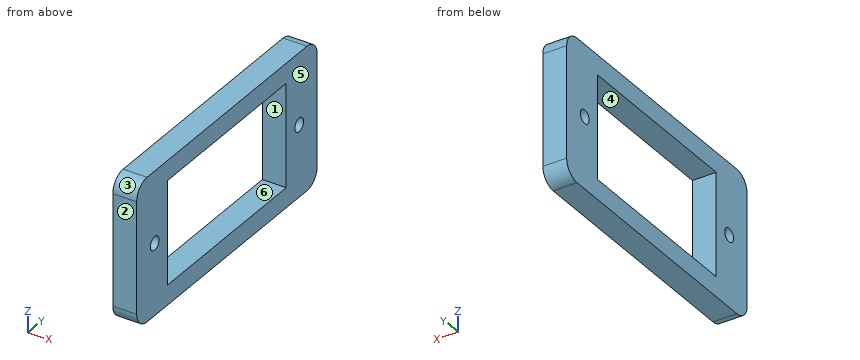
```python
from build123d import *

# Parameters (mm, degrees)
ESBO_O1_W                = 18
ESBO_O1_H                = 35
RESSALTO_EXTRUS_O1_DEPTH = 3
CORTE_EXTRUS_O1_REACH    = 21.906
ESBO_O2_W                = 13
ESBO_O2_H                = 23
CORTE_EXTRUS_O2_REACH    = 21.906
ESBO_O3_R                = 0.85
FILETE1_R                = 2


with BuildPart() as part:
    # Esboço1 → Ressalto-extrusão1 (new body)
    with BuildSketch(Plane(origin=(0, 0, 0), x_dir=(0, 0, -1), z_dir=(1, 0, 0))):
        Rectangle(ESBO_O1_W, ESBO_O1_H)
    extrude(amount=RESSALTO_EXTRUS_O1_DEPTH)

    # Esboço2 → Corte-extrusão1 (cut, up to next)
    with BuildSketch(Plane(origin=(3, 0, 0), x_dir=(0, 0, -1), z_dir=(1, 0, 0)), mode=Mode.PRIVATE) as corte_extrus_o1_sk1:
        Rectangle(ESBO_O2_W, ESBO_O2_H)
    corte_extrus_o1_tool1 = extrude(corte_extrus_o1_sk1.sketch, amount=-CORTE_EXTRUS_O1_REACH, mode=Mode.PRIVATE) & part.part
    add(corte_extrus_o1_tool1.solids().sort_by_distance((3, 0, 0))[0], mode=Mode.SUBTRACT)

    # Esboço3 → Corte-extrusão2 (cut, up to next)
    with BuildSketch(Plane.ZY, mode=Mode.PRIVATE) as corte_extrus_o2_sk1:
        with Locations((0, 14)):
            Circle(ESBO_O3_R)
    corte_extrus_o2_tool1 = extrude(corte_extrus_o2_sk1.sketch, amount=-CORTE_EXTRUS_O2_REACH, mode=Mode.PRIVATE) & part.part
    # Esboço3 → Corte-extrusão2 (cut, up to next)
    with BuildSketch(Plane.ZY, mode=Mode.PRIVATE) as corte_extrus_o2_sk2:
        with Locations((0, -14)):
            Circle(ESBO_O3_R)
    corte_extrus_o2_tool2 = extrude(corte_extrus_o2_sk2.sketch, amount=-CORTE_EXTRUS_O2_REACH, mode=Mode.PRIVATE) & part.part
    add(corte_extrus_o2_tool1.solids().sort_by_distance((0, 14, 0))[0], mode=Mode.SUBTRACT)
    add(corte_extrus_o2_tool2.solids().sort_by_distance((0, -14, 0))[0], mode=Mode.SUBTRACT)

    # Filete1
    filete1_edges = [part.edges().sort_by_distance(p)[0] for p in [
        (1.5, -17.5, -9),
        (1.5, -17.5, 9),
        (1.5, 17.5, 9),
        (1.5, 17.5, -9),
    ]]
    fillet(filete1_edges, radius=FILETE1_R)


solid = part.part
```
Geometry: final body of the model. Coordinates: model frame, mm. Face numbers are marked on the shaded views. A direction names the side the tool comes from. Give positions to 0.01 mm unless a question says otherwise; leave off trailing zeros. Loops run counter-clockwise (first coordinate to the right, second up) from the corner with the lowest first, then second, coordinate; pieces in that order, holes last. Notation, with made-up numbers: (-23.75, -31.5) -> (30.25, -31.5) arc R28 cw to (30.25, -13.5) -> close; hole circle Ø3 at (12.25, 69.5). An arc over 180 degrees is marked (long way). Use CSV: the item, a comma, the result in double quotes.
(1) Access query for the marked faces 1 and 2. Directions: +Z, -Z, +X, -X, +Y, -Y. A direction counts if a zero-diameter tool reaches every point of the face in a straight line with its end or side. Return the directions, or none.
From the geometry:
face 1,"+X, -X"
face 2,"+Z, -Z, +X, -X, -Y"
(2) First-contact query: P1, Ø4, axis at y = 8, z = 1.5, coming from the -X side. Flat tip, straight axial feed; report the tip coordinate or a pass-through.
From the geometry:
P1,"through"
(3) Cut plane C-C (y = 14). Output: boundary loops of the cut face in (x, z), plus the area to 3 significant figures.
From the geometry:
outline,"(0, -9) -> (3, -9) -> (3, -0.85) -> (0, -0.85) -> close; (0, 0.85) -> (3, 0.85) -> (3, 9) -> (0, 9) -> close"
area,"48.9 mm^2"
(4) Cut plane B-B (x = 0.9). Output: boundary loops of the cut face in (y, z), plus the area to 3 significant figures.
From the geometry:
outline,"(-17.5, -7) arc R2 ccw to (-15.5, -9) -> (15.5, -9) arc R2 ccw to (17.5, -7) -> (17.5, 7) arc R2 ccw to (15.5, 9) -> (-15.5, 9) arc R2 ccw to (-17.5, 7) -> close; hole circle Ø1.7 at (-14, 0); hole (-11.5, -6.5) -> (11.5, -6.5) -> (11.5, 6.5) -> (-11.5, 6.5) -> close; hole circle Ø1.7 at (14, 0)"
area,"323 mm^2"
(5) Pull-direction query (Y, two-part tool) for the marked faces 3, 4, 5 and 6; classes: released by +Y, released by -Y, zero draft, split by the parting line, or undercut.
From the geometry:
face 3,"released by -Y"
face 4,"undercut"
face 5,"zero draft"
face 6,"undercut"
(6) Cut plane A-A (z = -4.75). Output: boundary loops of the cut face in (x, y).
From the geometry:
outline,"(0, -17.5) -> (3, -17.5) -> (3, -11.5) -> (0, -11.5) -> close; (0, 11.5) -> (3, 11.5) -> (3, 17.5) -> (0, 17.5) -> close"
(7) Cut plane D-D (z = 0). Output: boundary loops of the cut face in (x, y).
From the geometry:
outline,"(0, -17.5) -> (3, -17.5) -> (3, -14.85) -> (0, -14.85) -> close; (0, -13.15) -> (3, -13.15) -> (3, -11.5) -> (0, -11.5) -> close; (0, 11.5) -> (3, 11.5) -> (3, 13.15) -> (0, 13.15) -> close; (0, 14.85) -> (3, 14.85) -> (3, 17.5) -> (0, 17.5) -> close"
(8) Ray query, line 1 along Y through (x, z) = (0.95, 0); line 2 along Y through (x, z) = (2.65, 0.75); line 3 along Y through (x, z) = (1.05, 1.25). Return the intervals inside material, ascending. Write a range as [from, to].
From the geometry:
line 1,"[-17.5, -14.85], [-13.15, -11.5], [11.5, 13.15], [14.85, 17.5]"
line 2,"[-17.5, -14.4], [-13.6, -11.5], [11.5, 13.6], [14.4, 17.5]"
line 3,"[-17.5, -11.5], [11.5, 17.5]"
